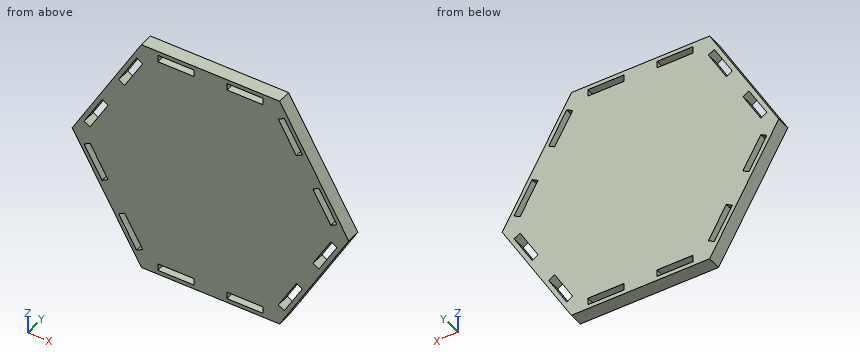
from build123d import *

# Parameters (mm, degrees)
BOSS_EXTRUDE1_DEPTH = 6.35
SKETCH2_W           = 16.51
SKETCH2_H           = 3.175
CUT_EXTRUDE1_DEPTH  = 7.35


with BuildPart() as part:
    # Sketch1 → Boss-Extrude1 (new body)
    with BuildSketch(Plane(origin=(0, 0, 0), x_dir=(1, 0, 0), z_dir=(0, 1, 0))):
        Polygon((-63.5, 0), (-31.75, -54.99261314), (31.75, -54.99261314), (63.5, 0), (31.75, 54.99261314), (-31.75, 54.99261314), align=None)
    extrude(amount=BOSS_EXTRUDE1_DEPTH)

    # Sketch2 → Cut-Extrude1 (cut, through all)
    with BuildSketch(Plane(origin=(0, 6.35, 0), x_dir=(1, 0, 0), z_dir=(0, 1, 0))):
        Polygon((-55.290590949, -4.059113577), (-58.040221606, -5.646613577), (-49.785221606, -19.944692993), (-47.035590949, -18.357192993), align=None)
        Polygon((-31.160590949, -45.853499563), (-33.910221606, -47.440999563), (-42.165221606, -33.142920147), (-39.415590949, -31.555420147), align=None)
        Polygon((-31.160590949, 45.853499563), (-33.910221606, 47.440999563), (-42.165221606, 33.142920147), (-39.415590949, 31.555420147), align=None)
        Polygon((-49.785221606, 19.944692993), (-47.035590949, 18.357192993), (-55.290590949, 4.059113577), (-58.040221606, 5.646613577), align=None)
        with Locations((15.875, 51.50011314)):
            Rectangle(SKETCH2_W, SKETCH2_H)
        with Locations((-15.875, 51.50011314)):
            Rectangle(SKETCH2_W, SKETCH2_H)
        Polygon((55.290590949, 4.059113577), (58.040221606, 5.646613577), (49.785221606, 19.944692993), (47.035590949, 18.357192993), align=None)
        Polygon((42.165221606, 33.142920147), (39.415590949, 31.555420147), (31.160590949, 45.853499563), (33.910221606, 47.440999563), align=None)
        Polygon((31.160590949, -45.853499563), (33.910221606, -47.440999563), (42.165221606, -33.142920147), (39.415590949, -31.555420147), align=None)
        Polygon((49.785221606, -19.944692993), (47.035590949, -18.357192993), (55.290590949, -4.059113577), (58.040221606, -5.646613577), align=None)
        with Locations((-15.875, -51.50011314)):
            Rectangle(SKETCH2_W, SKETCH2_H)
        with Locations((15.875, -51.50011314)):
            Rectangle(SKETCH2_W, SKETCH2_H)
    extrude(amount=-CUT_EXTRUDE1_DEPTH, mode=Mode.SUBTRACT)


solid = part.part
The model under review builds one solid part; all positions refer to its coordinate system, in mm. Round coordinates to 2 decimals unless told otherwise and drop trailing zeros. Loops run counter-clockwise (first coordinate to the right, second up) from the corner with the lowest first, then second, coordinate; pieces in that order, holes last. Notation, with made-up numbers: (66, 70.25) -> (105, 70.25) arc R8 cw to (105, 76.25) -> close; hole circle Ø1 at (82, -39.5). An arc over 180 degrees is marked (long way). Write item = value, one per line. Start each with the question number.
Item 1: Take a section at B-B on z = 39.5. Give the boundary of the cut face in (x, y), plus the area to 3 significant figures.
Item 2: Insertion check: pin 1 (3 mm diameter, centred on y = 2.5, z = -33, fed in from -X); pin 2 (2.5 mm diameter, centred on y = 4, z = -51.5, fed in from +X); pin 3 (1 mm diameter, centred on y = 3, z = -52, fed in from +X). Each pin has a flat end and moves straight along its axis. Give the tip position at first contact, or say it passes through.
Item 3: Take a section at C-C on y = 1. Count the separate pieces of the cut face and the enclosed holes in it, plus the area to 3 significant figures.
Item 4: To check wall thickness, follow L1, parallel to Z at x = -19.5, y = 2.5; L2, parallel to X at y = 5.75, z = -32.5; L3, parallel to Z at x = 35, y = 5.25. State the ranges of each line that lie inside material, in increasing order.
Item 5: Take a section at A-A on x = 21. Give the boundary of the cut face in (y, z).
Result:
q1.outline = (-40.69, 0) -> (-38.49, 0) -> (-38.49, 6.35) -> (-40.69, 6.35) -> close; (-34.83, 0) -> (34.83, 0) -> (34.83, 6.35) -> (-34.83, 6.35) -> close; (38.49, 0) -> (40.69, 0) -> (40.69, 6.35) -> (38.49, 6.35) -> close
q1.area = 470 mm²
q2.pin_1 = -45.31
q2.pin_2 = 34.49
q2.pin_3 = 33.77
q3.separate_pieces = 1
q3.enclosed_holes = 12
q3.area = 9,850 mm²
q4.L1 = -54.99 to -53.09, -49.91 to 49.91, 53.09 to 54.99
q4.L2 = -44.74 to -41.05, -38.87 to 38.87, 41.05 to 44.74
q4.L3 = -49.36 to -45.55, -39.2 to 39.2, 45.55 to 49.36
q5.outline = (0, -54.99) -> (6.35, -54.99) -> (6.35, -53.09) -> (0, -53.09) -> close; (0, -49.91) -> (6.35, -49.91) -> (6.35, 49.91) -> (0, 49.91) -> close; (0, 53.09) -> (6.35, 53.09) -> (6.35, 54.99) -> (0, 54.99) -> close
